from build123d import *

# Parameters (mm, degrees)
F0_R      = 12.5
F0_R_2    = 7.5
F1_DEPTH  = 28
F2_W      = 3.5
F2_H      = 7.3783658981
F5_R      = 8.5
F6_DEPTH  = 5
F9_DEPTH  = 30
F10_DEPTH = 25
F12_START = -5.8
F11_R     = 4
F12_DEPTH = 19.2


with BuildPart() as f1:
    # F0 (on Front) → F1 (new body)
    with BuildSketch(Plane.XZ):
        Circle(F0_R)
        Circle(F0_R_2, mode=Mode.SUBTRACT)
    extrude(amount=F1_DEPTH)

    # F2 (on Right) → F3 (revolve, cut)
    with BuildSketch(Plane.YZ):
        with Locations((-23.25, 6.2108170509)):
            Rectangle(F2_W, F2_H)
        with Locations((-4.75, 6.2108170509)):
            Rectangle(F2_W, F2_H)
    revolve(axis=Axis((0, -29.1106614321, 0), (0, 1, 0)), mode=Mode.SUBTRACT)

    # F5 (on mid) → F6 (join, symmetric)
    with BuildSketch(Plane.XZ.offset(14)):
        Circle(F5_R)
    extrude(amount=F6_DEPTH, both=True)

    # F8 (on face) → F9 (cut)
    with BuildSketch(Plane.XZ.offset(28)):
        with BuildLine():
            Line((0, 12.5), (0, 7.5))
            ThreePointArc((0, 7.5), (5.3033008589, 5.3033008589), (7.5, 0))
            ThreePointArc((7.5, 0), (5.3033008589, -5.3033008589), (0, -7.5))
            Line((0, -7.5), (0, -12.5))
            ThreePointArc((0, -12.5), (8.8388347648, -8.8388347648), (12.5, 0))
            ThreePointArc((12.5, 0), (8.8388347648, 8.8388347648), (0, 12.5))
        make_face()
        with BuildLine():
            Line((0, 7.5), (0, -2.1648029558))
            Line((0, -2.1648029558), (0, -7.5))
            ThreePointArc((0, -7.5), (5.3033008589, -5.3033008589), (7.5, 0))
            ThreePointArc((7.5, 0), (5.3033008589, 5.3033008589), (0, 7.5))
        make_face()
    extrude(amount=-F9_DEPTH, mode=Mode.SUBTRACT)

    # F7 (on Right) → F10 (cut)
    with BuildSketch(Plane.YZ):
        with BuildLine():
            ThreePointArc((-11.9, -8), (-12.5150757595, -6.5150757595), (-14, -5.9))
            ThreePointArc((-14, -5.9), (-15.4849242405, -9.4849242405), (-11.9, -8))
        make_face()
        with BuildLine():
            ThreePointArc((-11.9, 8), (-15.4849242405, 9.4849242405), (-14, 5.9))
            ThreePointArc((-14, 5.9), (-12.5150757595, 6.5150757595), (-11.9, 8))
        make_face()
    extrude(amount=-F10_DEPTH, mode=Mode.SUBTRACT)

    # F11 (on Right) → F12 (cut)
    with BuildSketch(Plane.YZ.offset(F12_START)):
        with Locations((-14, -8)):
            Circle(F11_R)
        with Locations((-14, 8)):
            Circle(F11_R)
    extrude(amount=-F12_DEPTH, mode=Mode.SUBTRACT)


solid = f1.part
CAD build for the part. Positions are in the model's coordinates, mm. A direction names the side the tool comes from. Round coordinates to 2 decimals unless told otherwise and drop trailing zeros. Order: outer loops, then holes, each group sorted by start corner. A loop starts at its lowest first (then second) coordinate and runs counter-clockwise, first axis right, second up. Notation, with made-up numbers: (12.5, 2) -> (67.5, 2) arc R11 cw to (67.5, 21) -> close; hole circle Ø1 at (69.5, 55.25). An arc over 180 degrees is marked (long way). Write each question's results on one line, items separated by ' | '.
1. Cut at D-D (z = -1). Give the cut face in (x, y), plus the area to 3 significant figures.
Findings below:
outline: (-12.46, -28) -> (-7.43, -28) -> (-7.43, -25) -> (-9.85, -25) -> (-9.85, -21.5) -> (-7.43, -21.5) -> (-7.43, -19) -> (0, -19) -> (0, -9) -> (-7.43, -9) -> (-7.43, -6.5) -> (-9.85, -6.5) -> (-9.85, -3) -> (-7.43, -3) -> (-7.43, 0) -> (-12.46, 0) -> close | area: 198 mm²
2. Wall check: line 1 along Y through (x, z) = (-1.25, -8); line 2 along Y through (x, z) = (-8, -2.25); line 3 along Z through (x, y) = (-2.7, -14). Give the ranges that are in metal, low to high. Write a range as [from, to].
Findings below:
line 1: y = [-28, -25], [-21.5, -16.1], [-11.9, -6.5], [-3, 0] | line 2: y = [-28, -25], [-21.5, -6.5], [-3, 0] | line 3: z = [-12.2, -10.1], [-5.9, 5.9], [10.1, 12.2]
3. 3-axis set-ups, long thin cutter, end or side, ignore diameter. For faces 1 (the face through (-8, 0, 0)), 2 (the face through (-3, -19, 0)), 3 (the face through (-8, -14, -4)), 4 (the face through (-7.5, -7.73, 0.16)), 5 (the face through (-9.898, -4.726, -0.218)): which of +Z, -Z, +X, -X, +Y, -Y reach the whole face in a straight line?
Findings below:
face 1: +Z, -Z, +X, -X, +Y | face 2: +X, -Y | face 3: -X | face 4: +X, +Y | face 5: +X
4. Flat gauge pins, fed straight in: P1, Ø10.5, axis at y = -14, z = -8, coming from the -X side; P2, Ø3.5, axis at y = -15, z = -7, coming from the -X side; P3, Ø1.5, axis at y = -13.5, z = -3, coming from the -X side. Where does each tip first touch, or does it go through?
Findings below:
P1: stops at x = -12.19 | P2: stops at x = -5.8 | P3: stops at x = -12.3
5. Cut at B-B (y = -15). Give the cut face in (x, z), plus the area to 3 significant figures.
Findings below:
outline: (-11.8, -4.13) -> (-5.8, -4.13) -> (-5.8, -6.15) -> (0, -6.15) -> (0, 6.15) -> (-5.8, 6.15) -> (-5.8, 4.13) -> (-11.8, 4.13) arc R12.5 ccw to start; (-5.8, -11.07) arc R12.5 ccw to (0, -12.5) -> (0, -9.85) -> (-5.8, -9.85) -> close; (-5.8, 9.85) -> (0, 9.85) -> (0, 12.5) arc R12.5 ccw to (-5.8, 11.07) -> close | area: 150 mm²
6. Pull direction Y, two halves, no side cores. Call faces 6 (the face through (-8, -28, 0)), 7 (the face through (-8, -14, 4)), 8 (the face through (-3, -9, 0)): pulls with the +Y half, pulls with the -Y half, needs draft (parallel to the pull), parting line crosses it, or undercut.
Findings below:
face 6: pulls with the -Y half | face 7: undercut | face 8: pulls with the +Y half
7. Cut at A-A (z = 9.5). Give the cut face in (x, y), plus the area to 3 significant figures.
Findings below:
outline: (-8.12, -28) -> (0, -28) -> (0, -25) -> (-2.79, -25) -> (-2.79, -21.5) -> (0, -21.5) -> (0, -15.47) -> (-5.8, -15.47) -> (-5.8, -17.71) -> (-8.12, -17.71) -> close; (-8.12, -10.29) -> (-5.8, -10.29) -> (-5.8, -12.53) -> (0, -12.53) -> (0, -6.5) -> (-2.79, -6.5) -> (-2.79, -3) -> (0, -3) -> (0, 0) -> (-8.12, 0) -> close | area: 174 mm²
8. Cut at C-C (x = -3.75). Count the separate pieces of the cut face and the enclosed holes in it, plus the area to 3 significant figures.
Findings below:
separate pieces: 1 | enclosed holes: 2 | area: 369 mm²
